```python
from build123d import *

# Parameters (mm, degrees)
F0_R     = 430
F1_DEPTH = 30
F2_R     = 385
F2_R_2   = 100
F3_DEPTH = 30
F4_DEPTH = 20


# Not quite as in the source:
# - a fillet or chamfer that OpenCascade refuses, or shapes differently, is made with other operations: its cross-section is extruded or revolved along the edge and cut away or added


with BuildPart() as f1:
    # F0 (on Front) → F1 (new body, symmetric)
    with BuildSketch(Plane.XZ):
        Circle(F0_R)
    extrude(amount=F1_DEPTH, both=True)

    # F2 (on face) → F3 (cut)
    with BuildSketch(Plane.XZ.offset(30)):
        Circle(F2_R)
        Circle(F2_R_2, mode=Mode.SUBTRACT)
    extrude(amount=-F3_DEPTH, mode=Mode.SUBTRACT)

    # F4 (add): a face of the model
    f4_faces = [f1.faces().sort_by_distance(p)[0] for p in [
        (0, -30, 0),
    ]]
    extrude(f4_faces, amount=F4_DEPTH)

    # F5: chamfer of 80 x 21.4359353945 on 1 edges, made by hand


with BuildPart() as f5_tool2:
    # F5_s3 → F5_t4 (revolve)
    with BuildSketch(Plane.XY):
        Polygon((121.4359353945, 0), (100, -80), (100, 0), align=None)
    revolve(axis=Axis((0, 0, 0), (0, -1, 0)))

    split(bisect_by=Plane.XZ.offset(50), keep=Keep.BOTTOM)


with BuildPart() as f1_1:
    add(f1.part)

    # F5_t1: union F5_tool2
    add(f5_tool2.part)

    # F6: chamfer of 30 x 39.0967611852 on 1 edges, made by hand


with BuildPart() as f6_tool2:
    # F6_s3 → F6_t4 (revolve)
    with BuildSketch(Plane.XY):
        Polygon((385, -39.0967611852), (355, 0), (385, 0), align=None)
    revolve(axis=Axis((0, 0, 0), (0, -1, 0)))

    split(bisect_by=Plane.XZ.offset(30), keep=Keep.BOTTOM)


with BuildPart() as f1_2:
    add(f1_1.part)

    # F6_t1: union F6_tool2
    add(f6_tool2.part)


solid = f1_2.part
```
Work out the finished part from the listing and answer in its coordinate system (mm). A direction names the side the tool comes from. Coordinates: 2 decimals unless noted, no trailing zeros. Write each loop counter-clockwise with the first axis right and the second up, starting at its lowest first coordinate (ties: lowest second). Pieces come first, ordered by that corner, then holes. Notation, with made-up numbers: (67.25, 8) - (84.25, 8) arc R25 ccw to (84.25, 35) - close; hole circle Ø5 at (10, 39.5). An arc over 180 degrees is marked (long way). Answer as a JSON object with one key per item and string values.
Q1. For a pull along X with two mould halves and no side action, classify faces 3 (the cylindrical face through (-341.23, -0.42, -261.65)), 4 (the flat face through (-2, -30, -380)), 5 (the conical face through (-77.2, -1.46, -347.65)) as pulls with the +X half, pulls with the -X half, needs draft (parallel to the pull), parting line crosses it, or undercut.
Results list:
{"face 3": "parting line crosses it", "face 4": "needs draft", "face 5": "undercut"}
Q2. Which of the six approach directions +Z, -Z, +X, -X, +Y, -Y give full straight-line access (tool end or side, diameter ignored) to faces 1 (the flat face through (153, 0, 5)), 2 (the flat face through (-6, 30, 6))?
Results list:
{"face 1": "-Y", "face 2": "+Z, -Z, +X, -X, +Y"}
Q3. Find section A-A (z = 0). Write down the section's boundary in (x, y).
Results list:
{"outline": "(-430, -30) - (-378.02, -30) - (-355, 0) - (-121.44, 0) - (-108.04, -50) - (108.04, -50) - (121.44, 0) - (355, 0) - (378.02, -30) - (430, -30) - (430, 30) - (-430, 30) - close"}
Q4. Find section C-C (y = 19). Write down the section's boundary in (x, z).
Results list:
{"outline": "circle Ø860 at (0, 0)"}
Q5. Consider L1, parallel to Y at x = 70, z = -194.5; L2, parallel to Y at x = -368.5, z = 129; L3, parallel to Z at x = 59, y = -23.5. Determine where each line is inside the solid, lowest interval first. Write a range as from..to.
Results list:
{"L1": "y = 0..30", "L2": "y = -30..30", "L3": "z = -425.93..-368.34, -98.87..98.87, 368.34..425.93"}
Q6. Given pin 1 Ø1 at (y, z) = (4.5, -239.5) entering from -X; pin 2 Ø1.5 at (y, z) = (6, 141.5) entering from +X; pin 3 Ø8 at (y, z) = (-31, -338.5) entering from -X, each flat-ended and moving along its own axis, determine where each tip first touches the part or whether it passes through.
Results list:
{"pin 1": "stops at x = -357.46", "pin 2": "stops at x = 406.31", "pin 3": "stops at x = -270.05"}
Q7. Find section B-B (x = 0). Write down the section's boundary in (y, z), plus the area to 3 significant figures.
Results list:
{"outline": "(-50, -108.04) - (0, -121.44) - (0, -355) - (-30, -378.02) - (-30, -430) - (30, -430) - (30, 430) - (-30, 430) - (-30, 378.02) - (0, 355) - (0, 121.44) - (-50, 108.04) - close", "area": "41,100 mm^2"}
